The figure shows three views and two pictorial views of one solid part (mm, origin at its lowest corner). Answer the questions. A direction names the side the tool comes from. Coordinates: 2 decimals unless noted, no trailing zeros. Order: outer loops, then holes, each group sorted by start corner. A loop starts at its lowest first (then second) coordinate and runs counter-clockwise, first axis right, second up. Notation, with made-up numbers: M -7.5,-12 L 20.5,-12 A21 cw 20.5,4 Z; hole C 54.25,65.5 d10. An arc over 180 degrees is marked long. Use a Markdown table: item, result.
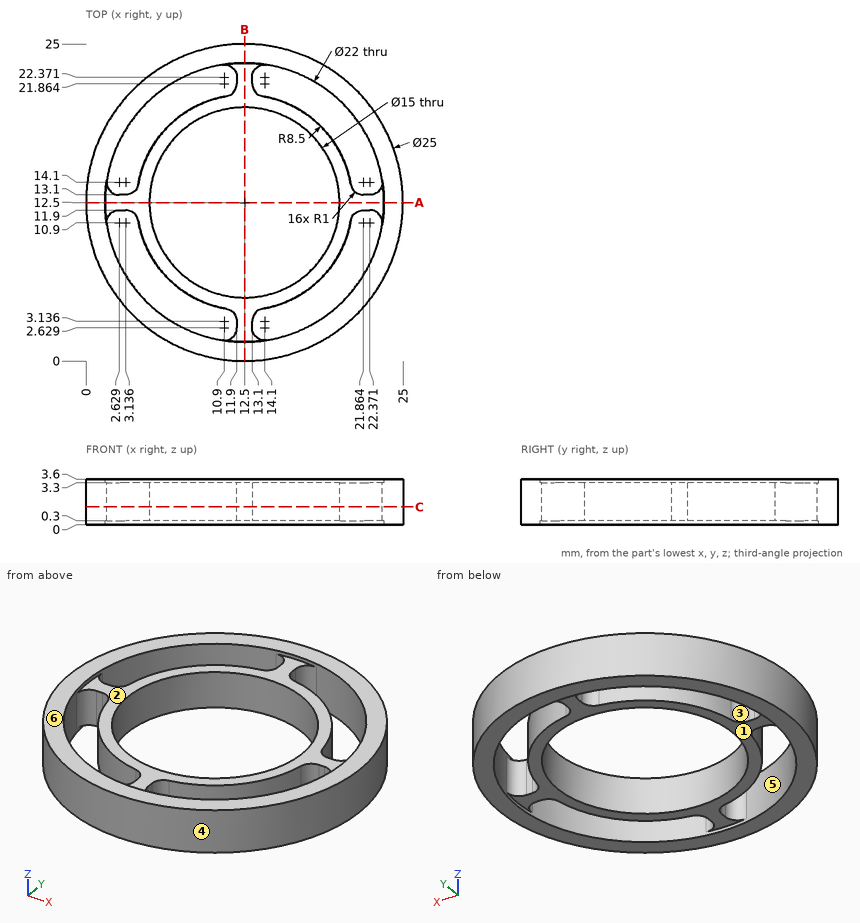
1. Find the intervals of material crossed by probe 1 along Y at (x, z) = (12.5, 2.7); probe 2 along Y at (x, z) = (15.5, 1.75) (1 decimal); probe 3 along X at (y, z) = (6.5, 1) (1 decimal), in increasing order.
Answers below:
| item | result |
|---|---|
| probe 1 | 0 to 5, 20 to 25 |
| probe 2 | 0.4 to 1.9, 4.5 to 5.6, 19.4 to 20.5, 23.1 to 24.6 |
| probe 3 | 1.5 to 3.3, 6.5 to 8, 17 to 18.5, 21.7 to 23.5 |
2. Section A-A on y = 12.5 is taken. Determine the outline of the cut face in (x, z), then the cut area to 3 significant figures.
Answers below:
| item | result |
|---|---|
| outline | M 0,0 L 1.5,0 L 1.5,0.3 L 5,0.3 L 5,3.3 L 1.5,3.3 L 1.5,3.6 L 0,3.6 Z; M 20,0.3 L 23.5,0.3 L 23.5,0 L 25,0 L 25,3.6 L 23.5,3.6 L 23.5,3.3 L 20,3.3 Z |
| area | 31.8 mm² |
3. For a pull along Y with two mould halves and no side action, classify the marked faces 4, 5 and 6 as +Y half, -Y half, draft (parallel to the pull), parting line (faces both ways), or undercut.
Answers below:
| item | result |
|---|---|
| face 4 | parting line |
| face 5 | undercut |
| face 6 | draft |
4. Flat-ended cylindrical pins translate along their axes: P1, Ø11, axis at x = 12.5, y = 14, coming from the +Z side; P2, Ø0.6, axis at x = 3, z = 1, coming from the -Y side; P3, Ø2, axis at y = 5.5, z = 2, coming from the +X side; P4, Ø5, axis at x = 5, y = 9, coming from the +Z side. Find the tip coordinate at first contact, or state that the pin passes through.
Answers below:
| item | result |
|---|---|
| P1 | through |
| P2 | y = 4.04 |
| P3 | x = 23.47 |
| P4 | z = 3.3 |
5. For the marked faces 1, 2 and 3, determine the directions among +Z, -Z, +X, -X, +Y, -Y from which every point of the face is accessible in a straight line to the end or side of a thin tool.
Answers below:
| item | result |
|---|---|
| face 1 | -Z |
| face 2 | +Z |
| face 3 | +Z, -Z |
6. Section C-C on z = 1.4 is taken. Give the number of separate pieces and of enclosed holes in the cut face.
Answers below:
| item | result |
|---|---|
| separate pieces | 1 |
| enclosed holes | 5 |
